Here's how the part is built. I have some questions about the finished solid (model axes, mm). A direction names the side the tool comes from. Give positions to 0.01 mm unless a question says otherwise; leave off trailing zeros. Order: outer loops, then holes, each group sorted by start corner. A loop starts at its lowest first (then second) coordinate and runs counter-clockwise, first axis right, second up.
from build123d import *

# Parameters (mm, degrees)
F0_W     = 670
F0_H     = 130
F1_DEPTH = 2100
F2_W     = 490.9612983465
F2_H     = 1275.4036784172
F3_DEPTH = 550
F4_W     = 670
F4_H     = 471.3955521584
F4_H_2   = 353.2007694244
F5_DEPTH = 500


with BuildPart() as f1:
    # F0 (on Front) → F1 (new body)
    with BuildSketch(Plane.XZ):
        Polygon((0, 402), (0, 0), (370, 0), (370, 82.8653350472), (370, 212.8653350472), (370, 402), align=None)
        with Locations((705, 147.8653350472)):
            Rectangle(F0_W, F0_H)
    extrude(amount=F1_DEPTH)

    # F2 (on face) → F3 (join)
    with BuildSketch(Plane(origin=(0, 0, 82.8653350472), x_dir=(1, 0, 0), z_dir=(0, 0, -1))):
        with Locations((388.9861777425, 1109.097391367)):
            Rectangle(F2_W, F2_H)
    extrude(amount=F3_DEPTH)

    # F4 (on face) → F5 (cut)
    with BuildSketch(Plane(origin=(0, 0, 82.8653350472), x_dir=(1, 0, 0), z_dir=(0, 0, -1))):
        with Locations((705, 235.6977760792)):
            Rectangle(F4_W, F4_H)
        with Locations((705, 1923.3996152878)):
            Rectangle(F4_W, F4_H_2)
    extrude(amount=-F5_DEPTH, mode=Mode.SUBTRACT)


solid = f1.part
Q1. If we section it at C-C on z = 262.5: List the corners of the cut face in (x, y) for me, plus the area to 3 significant figures.
Filled sheet:
outline: (0, -2100) - (370, -2100) - (370, 0) - (0, 0) - close
area: 777,000 mm2
Q2. For faces 1 (the face through (834, -1100, 82.865)), 2 (the face through (143.506, -1100, -230)), 3 (the face through (700, -1100, 212.865)), which set-ups out of +Z, -Z, +X, -X, +Y, -Y let a thin tool reach every point of the face, with its end or its side?
Filled sheet:
face 1: -Z, +X, +Y, -Y
face 2: -Z, -X, +Y, -Y
face 3: +Z, +X, +Y, -Y
Q3. If we section it at A-A on y = -936: List the corners of the cut face in (x, z) for me.
Filled sheet:
outline: (0, 0) - (143.51, 0) - (143.51, -467.13) - (634.47, -467.13) - (634.47, 82.87) - (1040, 82.87) - (1040, 212.87) - (370, 212.87) - (370, 402) - (0, 402) - close
Q4. If we section it at B-B on x = 825.5: List the corners of the cut face in (y, z) for me.
Filled sheet:
outline: (-1746.8, 82.87) - (-471.4, 82.87) - (-471.4, 212.87) - (-1746.8, 212.87) - close
Q5. I need wall thicknesses on L1, parallel to Z at x = 613, y = -750; L2, parallel to Y at x = 628, z = -236.5; L3, parallel to Z at x = 70.5, y = -417. Which ranges of each line are inside material? Lowest first, please.
Filled sheet:
L1: z = -467.13 to 212.87
L2: y = -1746.8 to -471.4
L3: z = 0 to 402
Q6. I'm going to push a flat-ended pin straight in: P1, Ø10, axis at x = 770.5, y = -681, coming from the +Z side. Where does the tip first touch, or does it pass through?
Filled sheet:
P1: stops at z = 212.87
